Source: CAD feature listing. Evaluate the final solid. Frame: model axes, mm. Face numbers are marked on the shaded views. A direction names the side the tool comes from. Give positions to 0.01 mm unless a question says otherwise; leave off trailing zeros. Write each loop counter-clockwise with the first axis right and the second up, starting at its lowest first coordinate (ties: lowest second). Pieces come first, ordered by that corner, then holes.
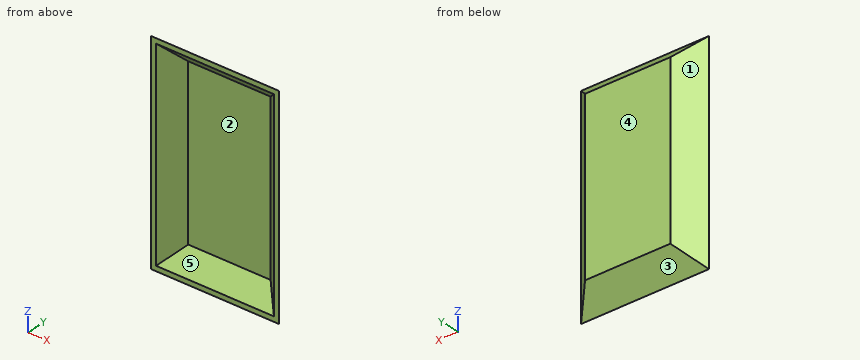
```python
from build123d import *

# Parameters (mm, degrees)
BOSS_EXTRUDE1_DEPTH     = 381
CUT_EXTRUDE1_DEPTH      = 451.805279472
CUT_EXTRUDE1_DEPTH_BACK = 451.805279472
SHELL2_T                = -12.7


with BuildPart() as part:
    # Sketch1 → Boss-Extrude1 (new, symmetric)
    with BuildSketch(Plane.XY):
        Polygon((-228.6, 0), (228.6, 0), (152.4, 76.2), (-152.4, 76.2), align=None)
    extrude(amount=BOSS_EXTRUDE1_DEPTH, both=True)

    # Sketch2 → Cut-Extrude1 (cut, two sides: drawn at the far end of the back side and taken through both)
    with BuildSketch(Plane(origin=(0, 0, 0), x_dir=(0, 0, -1), z_dir=(1, 0, 0)).offset(-CUT_EXTRUDE1_DEPTH_BACK)):
        Polygon((-381, 0), (-381, 76.2), (-304.8, 76.2), align=None)
        Polygon((381, 0), (381, 76.2), (304.8, 76.2), align=None)
    extrude(amount=CUT_EXTRUDE1_DEPTH + CUT_EXTRUDE1_DEPTH_BACK, mode=Mode.SUBTRACT)

    # Shell2
    shell2_openings = [part.faces().sort_by_distance(p)[0] for p in [
        (0, 0, 0),
    ]]
    offset(amount=SHELL2_T, openings=shell2_openings, kind=Kind.INTERSECTION)


solid = part.part
```
1. Section query C-C (y = 37.5). Return loops of the section in (x, z), plus the area to 3 significant figures.
2. Section query A-A (z = -282). Return loops of the section in (x, y).
3. Pull-direction query (Z, two-part tool) for the marked faces 1, 2 and 3; classes: pulls with the +Z half, pulls with the -Z half, needs draft (parallel to the pull), parting line crosses it, or undercut.
4. Section query B-B (x = -138.5). Return loops of the section in (y, z).
5. Line query: probe 1 along Z at (x, y) = (-11.5, 22.5); probe 2 along Y at (x, z) = (-127, -13.5); probe 3 along X at (y, z) = (32, 208). Output: solid intervals per line, ascending.
6. Access query for the marked faces 4 and 5. Directions: +Z, -Z, +X, -X, +Y, -Y. A direction counts if a zero-diameter tool reaches every point of the face in a straight line with its end or side. Return the directions, or none.
7. Pin query (flat end, axial travel): P1, Ø4, axis at x = -180, z = -25, coming from the +Y side; P2, Ø6, axis at x = -41.5, z = 10.5, coming from the -Y side; P3, Ø2, axis at y = 17.5, z = -88.5, coming from the +X side. Return the tip coordinate at first contact, or that it passes through.
The answers:
1. outline: (-191.1, -343.5) - (191.1, -343.5) - (191.1, 343.5) - (-191.1, 343.5) - close; hole (-173.14, -325.54) - (173.14, -325.54) - (173.14, 325.54) - (-173.14, 325.54) - close
1. area: 37,100 mm2
2. outline: (-228.6, 0) - (-210.64, 0) - (-147.14, 63.5) - (147.14, 63.5) - (210.64, 0) - (228.6, 0) - (152.4, 76.2) - (-152.4, 76.2) - close
3. face 1: needs draft
3. face 2: undercut
3. face 3: pulls with the -Z half
4. outline: (0, -381) - (76.2, -304.8) - (76.2, 304.8) - (0, 381) - (0, 363.04) - (63.5, 299.54) - (63.5, -299.54) - (0, -363.04) - close
5. probe 1: z = -358.5 to -340.54, 340.54 to 358.5
5. probe 2: y = 63.5 to 76.2
5. probe 3: x = -196.6 to -178.64, 178.64 to 196.6
6. face 4: +Z, -Z, +X, -X, +Y
6. face 5: -Y
7. P1: stops at y = 50.6
7. P2: stops at y = 63.5
7. P3: stops at x = 212.1
